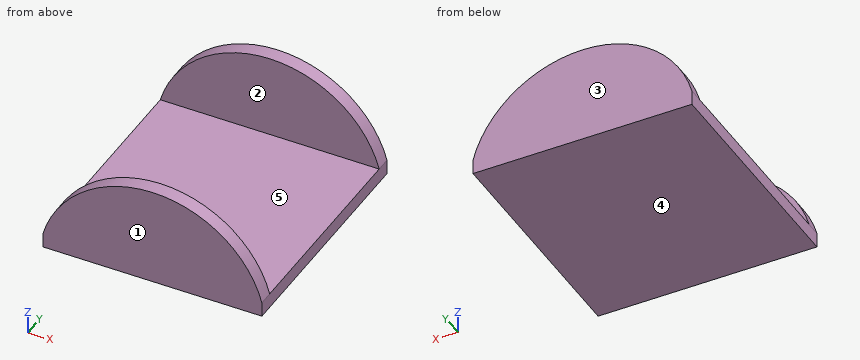
from build123d import *

# Parameters (mm, degrees)
BOSS_EXTRUDE1_DEPTH      = 5.08
BOSS_EXTRUDE2_DEPTH      = 76.2
BOSS_EXTRUDE2_DEPTH_BACK = 5.08
SKETCH3_W                = 74.93
SKETCH3_H                = 5.08
BOSS_EXTRUDE3_START      = -5.08
BOSS_EXTRUDE3_DEPTH      = 5.08


with BuildPart() as part:
    # Sketch2 → Boss-Extrude1 (new body)
    with BuildSketch(Plane(origin=(0, 0, 0), x_dir=(1, 0, 0), z_dir=(0, 1, 0))):
        with BuildLine():
            Line((-37.465, 0), (37.465, 0))
            ThreePointArc((37.465, 0), (0, -28.658189358), (-37.465, 0))
        make_face()
    extrude(amount=BOSS_EXTRUDE1_DEPTH)

    # Sketch3 → Boss-Extrude2 (add, two sides: drawn at the far end of the back side and taken through both)
    with BuildSketch(Plane(origin=(0, 5.08, 0), x_dir=(1, 0, 0), z_dir=(0, 1, 0)).offset(-BOSS_EXTRUDE2_DEPTH_BACK)):
        with Locations((0, 2.54)):
            Rectangle(SKETCH3_W, SKETCH3_H)
    extrude(amount=BOSS_EXTRUDE2_DEPTH + BOSS_EXTRUDE2_DEPTH_BACK)

    # Sketch4 → Boss-Extrude3 (add)
    with BuildSketch(Plane(origin=(0, 81.28, 0), x_dir=(1, 0, 0), z_dir=(0, 1, 0)).offset(BOSS_EXTRUDE3_START)):
        with BuildLine():
            Line((-37.465, 0), (37.465, 0))
            ThreePointArc((37.465, 0), (0, -28.658189358), (-37.465, 0))
        make_face()
    extrude(amount=BOSS_EXTRUDE3_DEPTH)


solid = part.part
Verification items for the finished model (mm, model axes). Face numbers are marked on the shaded views. A direction names the side the tool comes from. Coordinates: 2 decimals unless noted, no trailing zeros. Order: outer loops, then holes, each group sorted by start corner. A loop starts at its lowest first (then second) coordinate and runs counter-clockwise, first axis right, second up. Notation, with made-up numbers: (56.25, 6.5) -> (85.25, 6.5) arc R24 ccw to (85.25, 18.5) -> close; hole circle Ø1 at (26, -29.75). An arc over 180 degrees is marked (long way). Put each result on its own line as item: value. Start each with the question number.
1. Cross-section at C-C, the plane y = 50. Record the boundary of the cut face in (x, z) (3 decimals).
2. Cross-section at D-D, the plane z = 23.5. Record the boundary of the cut face in (x, y), then the cut area to 3 significant figures.
3. Material ranges on L1, parallel to Y at x = 25.5, z = 15; L2, parallel to Z at x = 23, y = 40; L3, parallel to X at y = 4, z = 16, recorded low to high. Write a range as [from, to].
4. Go/stop test with flat-tipped pins: pin 1 Ø21.5 at (x, y) = (-6, 49.5) entering from +Z; pin 2 Ø1 at (x, z) = (9.5, 15) entering from -Y. Record where each tip stops, or that it passes through.
5. Cross-section at A-A, the plane z = 11.5. Record the boundary of the cut face in (x, y).
6. Mould release check, pull along Y, two halves, no side actions. Record for the marked faces 1, 2 and 3: released by +Y, released by -Y, zero draft, split by the parting line, or undercut.
7. Access from +Z, -Z, +X, -X, +Y, -Y to the whole of each face (thin tool, end or side, straight path). Record for the marked faces 4 and 5.
8. Cross-section at B-B, the plane x = -31.5. Record the boundary of the cut face in (y, z).
Computed:
1. outline: (-37.465, -5.08) -> (37.465, -5.08) -> (37.465, 0) -> (-37.465, 0) -> close
2. outline: (-19.34, 0) -> (19.34, 0) -> (19.34, 5.08) -> (-19.34, 5.08) -> close; (-19.34, 76.2) -> (19.34, 76.2) -> (19.34, 81.28) -> (-19.34, 81.28) -> close
2. area: 393 mm2
3. L1: [0, 5.08], [76.2, 81.28]
3. L2: [-5.08, 0]
3. L3: [-28.68, 28.68]
4. pin 1: z = 0
4. pin 2: y = 0
5. outline: (-32.21, 0) -> (32.21, 0) -> (32.21, 5.08) -> (-32.21, 5.08) -> close; (-32.21, 76.2) -> (32.21, 76.2) -> (32.21, 81.28) -> (-32.21, 81.28) -> close
6. face 1: released by -Y
6. face 2: undercut
6. face 3: released by +Y
7. face 4: -Z, +X, -X, +Y, -Y
7. face 5: +Z, +X, -X
8. outline: (0, -5.08) -> (81.28, -5.08) -> (81.28, 12.52) -> (76.2, 12.52) -> (76.2, 0) -> (5.08, 0) -> (5.08, 12.52) -> (0, 12.52) -> close
